Geometry: final body of the model. Coordinates: model frame, mm. A direction names the side the tool comes from. Round coordinates to 2 decimals unless told otherwise and drop trailing zeros. Loops run counter-clockwise (first coordinate to the right, second up) from the corner with the lowest first, then second, coordinate; pieces in that order, holes last. Notation, with made-up numbers: (1, -38.75) - (21, -38.75) arc R33 cw to (21, -6.75) - close; hole circle Ø8 at (19, 77.5). An arc over 180 degrees is marked (long way). Write item = value, one per line. Start each with the question number.
Item 1: Access query for faces 1 (the flat face through (7.9, 0, -32)), 2 (the flat face through (6, -6.8, -42)), 3 (the flat face through (6, 7.45, -41)). Directions: +Z, -Z, +X, -X, +Y, -Y. A direction counts if a zero-diameter tool reaches every point of the face in a straight line with its end or side. Return the directions, or none.
Item 2: Section C-C (z = -32). Return loops of the section in (x, y), plus the area to 3 significant figures.
Item 3: First-contact query: pin 1 (1.5 mm diameter, centred on x = -7.5, z = -6.5, fed in from -Y); pin 2 (0.6 mm diameter, centred on x = -6.5, z = -40.5, fed in from +Y); pin 3 (1 mm diameter, centred on x = 6.5, z = -41.5, fed in from -Y); pin 4 (12.5 mm diameter, centred on x = -3.5, y = -1.5, fed in from -Z). Flat tips, straight axial feed; report the tip coordinate or a pass-through.
Item 4: Draft query along X for faces 4 (the flat face through (0, 9, -32)), 5 (the flat face through (5.515, -6, -40)), 6 (the flat face through (-6.785, 6, -40)). Return one class per face: pulls with the +X half, pulls with the -X half, needs draft (parallel to the pull), parting line crosses it, or undercut.
Item 5: Section A-A (y = -6.05). Count the separate pieces of the cut face and the enclosed holes in it, plus the area to 3 significant figures.
Item 6: Section B-B (z = -5.5). Return loops of the section in (x, y).
Item 7: Line query: line 1 (Y direction, x = 4.5, z = -27.5); line 2 (X direction, y = 5, z = -31.5); line 3 (Y direction, x = -11, z = -7.5). Output: solid intervals per line, ascending. Write a range as from..to.
from build123d import *

# Parameters (mm, degrees)
SKETCH2_W           = 15.8
SKETCH2_H           = 18
BOSS_EXTRUDE2_DEPTH = 11.2
SKETCH3_W           = 1.27
SKETCH3_H           = 6.5
BOSS_EXTRUDE3_DEPTH = 18
SKETCH4_W           = 6.5
SKETCH4_H           = 1.55
SKETCH4_H_2         = 9.3
CUT_EXTRUDE1_DEPTH  = 52.337960929
CUT_EXTRUDE2_DEPTH  = 52.337960929


with BuildPart() as part:
    # Sketch1 → Revolve1 (revolve)
    with BuildSketch(Plane(origin=(0, 0, 0), x_dir=(0, 0, -1), z_dir=(1, 0, 0)), mode=Mode.PRIVATE) as revolve1_sk:
        with BuildLine():
            Line((0, 15), (1.5, 15))
            Line((1.5, 15), (2.5, 14))
            Line((2.5, 14), (8.5, 14))
            Line((8.5, 14), (9.5, 12))
            Line((9.5, 12), (11.5, 12))
            Line((11.5, 12), (11.5, 11))
            Line((11.5, 11), (15.5, 11))
            Line((15.5, 11), (15.5, 8))
            Line((15.5, 8), (26.3, 8))
            Line((26.3, 8), (26.3, 0))
            Line((26.3, 0), (-4.5, 0))
            add(Edge.make_bspline(
                [(-4.5, 0), (-4.300353952, 5.255228693), (-2.977309479, 10.604163614), (0, 15)],
                knots=[0, 0, 0, 0, 1, 1, 1, 1], degree=3))
        make_face()
    revolve(revolve1_sk.sketch.rotate(Axis((0, 0, 0), (0, 0, -1)), 90), axis=Axis((0, 0, 0), (0, 0, -1)))

    # Sketch2 → Boss-Extrude2 (add)
    with BuildSketch(Plane(origin=(0, 0, -26.3), x_dir=(-1, 0, 0), z_dir=(0, 0, -1))):
        Rectangle(SKETCH2_W, SKETCH2_H)
    extrude(amount=BOSS_EXTRUDE2_DEPTH)

    # Sketch3 → Boss-Extrude3 (add)
    with BuildSketch(Plane(origin=(0, 9, 0), x_dir=(1, 0, 0), z_dir=(0, 1, 0))):
        with Locations((-6.15, 40.75)):
            Rectangle(SKETCH3_W, SKETCH3_H)
        with Locations((6.15, 40.75)):
            Rectangle(SKETCH3_W, SKETCH3_H)
    extrude(amount=-BOSS_EXTRUDE3_DEPTH)

    # Sketch4 → Cut-Extrude1 (cut, through all)
    with BuildSketch(Plane(origin=(6.785, 0, 0), x_dir=(0, 0, -1), z_dir=(1, 0, 0))):
        with Locations((40.75, 8.225)):
            Rectangle(SKETCH4_W, SKETCH4_H)
        with Locations((40.75, 0)):
            Rectangle(SKETCH4_W, SKETCH4_H_2)
        with Locations((40.75, -8.225)):
            Rectangle(SKETCH4_W, SKETCH4_H)
    extrude(amount=-CUT_EXTRUDE1_DEPTH, mode=Mode.SUBTRACT)

    # Sketch5 → Cut-Extrude2 (cut, through all)
    with BuildSketch(Plane(origin=(6.785, 0, 0), x_dir=(0, 0, -1), z_dir=(1, 0, 0))):
        with BuildLine():
            Line((41.1, 6.8), (42.5, 6.8))
            ThreePointArc((42.5, 6.8), (43.25, 6.05), (42.5, 5.3))
            Line((42.5, 5.3), (41.1, 5.3))
            ThreePointArc((41.1, 5.3), (40.35, 6.05), (41.1, 6.8))
        make_face()
    cut_extrude2 = extrude(amount=-CUT_EXTRUDE2_DEPTH, mode=Mode.SUBTRACT)

    # Mirror1: Cut-Extrude2 across plane
    add(cut_extrude2.mirror(Plane.ZX), mode=Mode.SUBTRACT)


solid = part.part
Taken from the geometry:
q1.face_1 = -Z, +X, +Y, -Y
q1.face_2 = +X, -X
q1.face_3 = -Z, +X, -X, +Y
q2.outline = (-7.9, -9) - (7.9, -9) - (7.9, 9) - (-7.9, 9) - close
q2.area = 284 mm^2
q3.pin_1 = -12.27
q3.pin_2 = 7.45
q3.pin_3 = -7.45
q3.pin_4 = -44
q4.face_4 = needs draft
q4.face_5 = undercut
q4.face_6 = pulls with the -X half
q5.separate_pieces = 3
q5.enclosed_holes = 0
q5.area = 726 mm^2
q6.outline = circle Ø28 at (0, 0)
q7.line_1 = -9..9
q7.line_2 = -7.9..7.9
q7.line_3 = -8.66..8.66
